Model file for the job. Use its own axes, mm. A direction names the side the tool comes from. Coordinates: 2 decimals unless noted, no trailing zeros. Order: outer loops, then holes, each group sorted by start corner. A loop starts at its lowest first (then second) coordinate and runs counter-clockwise, first axis right, second up. Notation, with made-up numbers: (74.25, 44.5) - (83.25, 44.5) arc R7 cw to (83.25, 57.5) - close; hole circle Ø5 at (73.25, 27.25). An arc over 180 degrees is marked (long way). Put each result on its own line as item: value. Start each with the question number.
```python
from build123d import *
from OCP.BRepFilletAPI import BRepFilletAPI_MakeChamfer

# Parameters (mm, degrees)
RESSALTO_EXTRUS_O1_DEPTH = 13
ESBO_O2_W                = 15
ESBO_O2_H                = 6
ESBO_O2_W_2              = 4
ESBO_O2_H_2              = 16
RESSALTO_EXTRUS_O2_DEPTH = 15
ESBO_O3_R                = 1
CORTE_EXTRUS_O1_DEPTH    = 77.870020164
ESBO_O10_R               = 1.7
CORTE_EXTRUS_O4_DEPTH    = 10
ESBO_O11_W               = 25
ESBO_O11_H               = 34.7
CORTE_EXTRUS_O5_DEPTH    = 10
RESSALTO_EXTRUS_O3_DEPTH = 17
RESSALTO_EXTRUS_O4_REACH = 77.374
ESBO_O7_W                = 4
ESBO_O7_H                = 5
ESBO_O8_W                = 15
ESBO_O8_H                = 3.5
RESSALTO_EXTRUS_O5_DEPTH = 2.5
CHANFRO2_SIZE            = 2
CHANFRO2_SIZE_2          = 7
CHANFRO3_SIZE            = 1.5
CHANFRO3_SIZE2           = 3.216760381
ESBO_O12_W               = 12.6
ESBO_O12_H               = 10.6
CORTE_EXTRUS_O6_DEPTH    = 10
CORTE_EXTRUS_O7_DEPTH    = 22
ESBO_O15_R               = 2
CORTE_EXTRUS_O9_DEPTH    = 15
ESBO_O17_W               = 15
ESBO_O17_H               = 35.3
CORTE_EXTRUS_O10_DEPTH   = 4
ESBO_O18_W               = 7.5
ESBO_O18_H               = 6
CORTE_EXTRUS_O11_DEPTH   = 11


with BuildPart() as part:
    # Esboço1 → Ressalto-extrusão1 (new body)
    with BuildSketch(Plane.XY):
        Polygon((-12.5, 0), (12.5, 0), (12.5, -40), (7.5, -70), (-7.5, -70), (-12.5, -40), align=None)
    extrude(amount=RESSALTO_EXTRUS_O1_DEPTH)

    # Esboço2 → Ressalto-extrusão2 (add)
    with BuildSketch(Plane.XY.offset(13)):
        with Locations((-5, -32.3)):
            Rectangle(ESBO_O2_W, ESBO_O2_H)
        with Locations((-5, -3)):
            Rectangle(ESBO_O2_W, ESBO_O2_H)
        with Locations((10.5, -12)):
            Rectangle(ESBO_O2_W_2, ESBO_O2_H_2)
    extrude(amount=RESSALTO_EXTRUS_O2_DEPTH)

    # Esboço3 → Corte-extrusão1 (cut, through all)
    with BuildSketch(Plane(origin=(2.5, 0, 0), x_dir=(0, 0, -1), z_dir=(1, 0, 0))):
        with Locations(Location((-20.5, -3.8, 0), (0, 0, 90))):
            Circle(ESBO_O3_R)
        with Locations(Location((-20.5, -31.5, 0), (0, 0, 270))):
            Circle(ESBO_O3_R)
    extrude(amount=-CORTE_EXTRUS_O1_DEPTH, mode=Mode.SUBTRACT)

    # Esboço10 → Corte-extrusão4 (cut)
    with BuildSketch(Plane(origin=(12.5, 0, 0), x_dir=(0, 0, -1), z_dir=(1, 0, 0))):
        with Locations((-20.5, -12)):
            Circle(ESBO_O10_R)
        with BuildLine():
            Line((-13, -4), (-28, -4))
            Line((-28, -4), (-28, -20))
            Line((-28, -20), (-13, -20))
            Line((-13, -20), (-21.684004699, -18.391254405))
            ThreePointArc((-21.684004699, -18.391254405), (-27, -12), (-21.684004699, -5.608745595))
            Line((-21.684004699, -5.608745595), (-13, -4))
        make_face()
    extrude(amount=-CORTE_EXTRUS_O4_DEPTH, mode=Mode.SUBTRACT)

    # Esboço11 → Corte-extrusão5 (cut)
    with BuildSketch(Plane.XY.offset(13)):
        with Locations((0, -52.65)):
            Rectangle(ESBO_O11_W, ESBO_O11_H)
    extrude(amount=-CORTE_EXTRUS_O5_DEPTH, mode=Mode.SUBTRACT)

    # Esboço6 → Ressalto-extrusão3 (add)
    with BuildSketch(Plane.XZ.offset(70)):
        Polygon((-5, 4), (-5, 7.5), (-4.75, 7.5), (-4.75, 10), (-7.5, 10), (-7.5, 3), (7.5, 3), (7.5, 10), (4.75, 10), (4.75, 7.5), (5, 7.5), (5, 4), align=None)
    extrude(amount=-RESSALTO_EXTRUS_O3_DEPTH)

    # Ressalto-extrusão4: up to this face of the body (flat: up to its plane)
    ressalto_extrus_o4_end = Plane(part.part.faces().sort_by_distance((-6.125, -61.5, 10))[0])
    # Esboço7 → Ressalto-extrusão4 (add, up to the picked face)
    with BuildSketch(Plane.XY.offset(3), mode=Mode.PRIVATE) as ressalto_extrus_o4_sk1:
        with Locations((0, -40.5)):
            Rectangle(ESBO_O7_W, ESBO_O7_H)
    ressalto_extrus_o4_tool1 = split(extrude(ressalto_extrus_o4_sk1.sketch, amount=RESSALTO_EXTRUS_O4_REACH, mode=Mode.PRIVATE), bisect_by=ressalto_extrus_o4_end, keep=Keep.BOTH, mode=Mode.PRIVATE)
    # Esboço7 → Ressalto-extrusão4 (add, up to the picked face)
    with BuildSketch(Plane.XY.offset(3), mode=Mode.PRIVATE) as ressalto_extrus_o4_sk2:
        with Locations((5.5, -55.5)):
            Rectangle(ESBO_O7_W, ESBO_O7_H)
    ressalto_extrus_o4_tool2 = split(extrude(ressalto_extrus_o4_sk2.sketch, amount=RESSALTO_EXTRUS_O4_REACH, mode=Mode.PRIVATE), bisect_by=ressalto_extrus_o4_end, keep=Keep.BOTH, mode=Mode.PRIVATE)
    # Esboço7 → Ressalto-extrusão4 (add, up to the picked face)
    with BuildSketch(Plane.XY.offset(3), mode=Mode.PRIVATE) as ressalto_extrus_o4_sk3:
        with Locations((-5.5, -55.5)):
            Rectangle(ESBO_O7_W, ESBO_O7_H)
    ressalto_extrus_o4_tool3 = split(extrude(ressalto_extrus_o4_sk3.sketch, amount=RESSALTO_EXTRUS_O4_REACH, mode=Mode.PRIVATE), bisect_by=ressalto_extrus_o4_end, keep=Keep.BOTH, mode=Mode.PRIVATE)
    add(ressalto_extrus_o4_tool1.solids().sort_by(Axis((0, -40.5, 3), (0, 0, 1)))[0])
    add(ressalto_extrus_o4_tool2.solids().sort_by(Axis((5.5, -55.5, 3), (0, 0, 1)))[0])
    add(ressalto_extrus_o4_tool3.solids().sort_by(Axis((-5.5, -55.5, 3), (0, 0, 1)))[0])

    # Esboço8 → Ressalto-extrusão5 (add)
    with BuildSketch(Plane.XY.offset(10)):
        with Locations((0, -68.25)):
            Rectangle(ESBO_O8_W, ESBO_O8_H)
        with Locations((0, -55.75)):
            Rectangle(ESBO_O8_W, ESBO_O8_H)
    extrude(amount=-RESSALTO_EXTRUS_O5_DEPTH)

    # Chanfro2
    chanfro2_edges_1 = [part.edges().sort_by_distance(p)[0] for p in [
        (7.5, -61.5, 3),
    ]]
    chanfro2_side_1 = [part.faces().sort_by_distance(p)[0] for p in [
        (7.54, -61.5, 3),
    ]]
    chanfro2_edges_2 = [part.edges().sort_by_distance(p)[0] for p in [
        (-7.5, -61.5, 3),
    ]]
    chanfro2_side_2 = [part.faces().sort_by_distance(p)[0] for p in [
        (-7.54, -61.5, 3),
    ]]
    chanfro2 = BRepFilletAPI_MakeChamfer(part.part.solid().wrapped)
    for e in chanfro2_edges_1:
        chanfro2.Add(CHANFRO2_SIZE - 0.0001, CHANFRO2_SIZE_2 - 0.0001, e.wrapped, chanfro2_side_1[0].wrapped)
    for e in chanfro2_edges_2:
        chanfro2.Add(CHANFRO2_SIZE - 0.0001, CHANFRO2_SIZE_2 - 0.0001, e.wrapped, chanfro2_side_2[0].wrapped)
    add(Compound.cast(chanfro2.Shape()), mode=Mode.REPLACE)  # a hair under: the kernel refuses the full size

    # Chanfro3
    chanfro3_edges = [part.edges().sort_by_distance(p)[0] for p in [
        (0, -70, 0),
    ]]
    chanfro3_side = [part.faces().sort_by_distance(p)[0] for p in [
        (7.319722436, -70, 9.99995),
    ]]
    chamfer(chanfro3_edges, length=CHANFRO3_SIZE, length2=CHANFRO3_SIZE2, reference=chanfro3_side[0])

    # Esboço12 → Corte-extrusão6 (cut)
    with BuildSketch(Plane(origin=(0, 0, 0), x_dir=(1, 0, 0), z_dir=(0, 1, 0))):
        with Locations((0, -6.5)):
            Rectangle(ESBO_O12_W, ESBO_O12_H)
    extrude(amount=-CORTE_EXTRUS_O6_DEPTH, mode=Mode.SUBTRACT)

    # Esboço13 → Corte-extrusão7 (cut)
    with BuildSketch(Plane(origin=(0, -10, 0), x_dir=(1, 0, 0), z_dir=(0, 1, 0))):
        with BuildLine():
            Line((-3.405877273, -11.8), (3.405877273, -11.8))
            ThreePointArc((3.405877273, -11.8), (6.3, -6.5), (3.405877273, -1.2))
            Line((3.405877273, -1.2), (-3.405877273, -1.2))
            ThreePointArc((-3.405877273, -1.2), (-6.3, -6.5), (-3.405877273, -11.8))
        make_face()
    extrude(amount=-CORTE_EXTRUS_O7_DEPTH, mode=Mode.SUBTRACT)

    # Esboço15 → Corte-extrusão9 (cut)
    with BuildSketch(Plane.ZY.offset(12.5)):
        with Locations((6, -28)):
            Circle(ESBO_O15_R)
    extrude(amount=-CORTE_EXTRUS_O9_DEPTH, mode=Mode.SUBTRACT)

    # Esboço17 → Corte-extrusão10 (cut)
    with BuildSketch(Plane.XY.offset(28)):
        with Locations((-5, -17.65)):
            Rectangle(ESBO_O17_W, ESBO_O17_H)
    extrude(amount=-CORTE_EXTRUS_O10_DEPTH, mode=Mode.SUBTRACT)

    # Esboço18 → Corte-extrusão11 (cut)
    with BuildSketch(Plane.XY.offset(24)):
        with Locations((-1.25, -3)):
            Rectangle(ESBO_O18_W, ESBO_O18_H)
    extrude(amount=-CORTE_EXTRUS_O11_DEPTH, mode=Mode.SUBTRACT)


solid = part.part
```
Item 1: Pull direction Z, two halves, no side cores. Call faces 1 (the face through (10.528, -19.207, 17.281)), 2 (the face through (0, -12, 1.2)), 3 (the face through (-2, -41, 6)), 4 (the face through (-6, -10, 2)): pulls with the +Z half, pulls with the -Z half, needs draft (parallel to the pull), parting line crosses it, or undercut.
Item 2: Flat gauge pins, fed straight in: pin 1 Ø6 at (x, z) = (8.5, 22.5) entering from +Y; pin 2 Ø1.8 at (x, y) = (-2.5, -33.5) entering from +Z; pin 3 Ø3 at (y, z) = (-64.5, 6.5) entering from -X. Where does each tip first touch, or does it go through?
Item 3: Slice it at B-B, the plane z = 20.5. Give the cut face in (x, y), plus the area to 3 significant figures.
Item 4: Slice it at D-D, the plane z = 9. Give the number of separate pieces and of enclosed holes in the cut face, plus the area to 3 significant figures.
Item 5: 3-axis set-ups, long thin cutter, end or side, ignore diameter. For faces 5 (the face through (-6.3, -20.8, 6.4)), 6 (the face through (0, -41, 10)), 7 (the face through (0, -17, 13)): which of +Z, -Z, +X, -X, +Y, -Y reach the whole face in a straight line?
Item 6: Slice it at A-A, the plane y = -12. Give the cut face in (x, z), plus the area to 3 significant figures.
Item 7: Wall check: line 1 along Z through (x, y) = (-3, -31.5); line 2 along Y through (x, z) = (-11, 6); line 3 along Y through (x, z) = (-8.75, 20.75). Give the ranges that are in metal, low to high.
Item 8: Slice it at C-C, the plane z = 16.5. Give the cut face in (x, y).
Here are the results:
1. face 1: pulls with the +Z half
1. face 2: undercut
1. face 3: needs draft
1. face 4: undercut
2. pin 1: stops at y = -5.2
2. pin 2: stops at z = 24
2. pin 3: stops at x = -8.65
3. outline: (-12.5, -35.3) - (2.5, -35.3) - (2.5, -32.5) - (-12.5, -32.5) - close; (-12.5, -30.5) - (2.5, -30.5) - (2.5, -29.3) - (-12.5, -29.3) - close; (-12.5, -6) - (-5, -6) - (-5, -4.8) - (-12.5, -4.8) - close; (-12.5, -2.8) - (-5, -2.8) - (-5, 0) - (-12.5, 0) - close; (8.5, -18.61) - (12.5, -18.61) - (12.5, -13.7) - (8.5, -13.7) - close; (8.5, -10.3) - (12.5, -10.3) - (12.5, -5.39) - (8.5, -5.39) - close
3. area: 129 mm^2
4. separate pieces: 3
4. enclosed holes: 1
4. area: 695 mm^2
5. face 5: +Y
5. face 6: +Z, +X, -X, -Y
5. face 7: +Z
6. outline: (-12.5, 0) - (12.5, 0) - (12.5, 18.8) - (8.5, 18.8) - (8.5, 13) - (-12.5, 13) - close; (8.5, 22.2) - (12.5, 22.2) - (12.5, 27) - (8.5, 27) - close; hole (-3.41, 1.2) - (3.41, 1.2) arc R6.3 ccw to (3.41, 11.8) - (-3.41, 11.8) arc R6.3 ccw to start
6. area: 252 mm^2
7. line 1: z = 0 to 1.2, 11.8 to 19.5, 21.5 to 24
7. line 2: y = -35.3 to -30, -26 to 0
7. line 3: y = -35.3 to -32.47, -30.53 to -29.3, -6 to -4.77, -2.83 to 0
8. outline: (-12.5, -35.3) - (2.5, -35.3) - (2.5, -29.3) - (-12.5, -29.3) - close; (-12.5, -6) - (-5, -6) - (-5, 0) - (-12.5, 0) - close; (8.5, -19.35) - (12.5, -19.35) - (12.5, -4.65) - (8.5, -4.65) - close
